Read the model definition and answer for the solid it produces. Units are mm, in the model's axes. A direction names the side the tool comes from. Round coordinates to 2 decimals unless told otherwise and drop trailing zeros. Order: outer loops, then holes, each group sorted by start corner. A loop starts at its lowest first (then second) coordinate and runs counter-clockwise, first axis right, second up. Notation, with made-up numbers: (89, -22) -> (114, -22) arc R21 cw to (114, -18) -> close; hole circle Ø9 at (32, -16.75). An arc over 180 degrees is marked (long way). Answer as a JSON object with one key per item and string values. Group by question number.
Item 1: Section B-B, the plane z = 10.5 is taken. Write down the section's boundary in (x, y), plus the area to 3 significant figures.
Item 2: Consider probe 1 along X at (y, z) = (1.5, -6); probe 2 along Y at (x, z) = (-2.75, 0.5). Determine where each line is inside the solid, lowest interval first. Write a range as from..to.
Item 3: The mould has two halves that part along X. Classify faces 3 (the flat face through (-6, -0.9, 0)), 4 (the flat face through (0, 2.4, 0)), 5 (the flat face through (3.5, 1, 0)), 6 (the flat face through (-8.5, 2, 0)): pulls with the +X half, pulls with the -X half, needs draft (parallel to the pull), parting line crosses it, or undercut.
Item 4: For faces 1 (the flat face through (-3.5, 1, 0)), 2 (the flat face through (0, 3, -15.4)), determine the directions among +Z, -Z, +X, -X, +Y, -Y from which every point of the face is accessible in a straight line to the end or side of a thin tool.
Item 5: Section A-A, the plane y = 0 is taken. Write down the section's boundary in (x, z), plus the area to 3 significant figures.
Item 6: Section C-C, the plane x = -2.25 is taken. Write down the section's boundary in (y, z).
from build123d import *

# Parameters (mm, degrees)
BOSS_EXTRUDE1_DEPTH = 15.4


with BuildPart() as part:
    # Sketch1 → Boss-Extrude1 (new, symmetric)
    with BuildSketch(Plane.XY):
        Polygon((3.5, 2.4), (3.5, -0.9), (8.5, -0.9), (8.5, 5.6), (-8.5, 5.6), (-8.5, -0.9), (-3.5, -0.9), (-3.5, 2.4), align=None)
    extrude(amount=BOSS_EXTRUDE1_DEPTH, both=True)


solid = part.part
Values found:
{
 "1": {"outline": "(-8.5, -0.9) -> (-3.5, -0.9) -> (-3.5, 2.4) -> (3.5, 2.4) -> (3.5, -0.9) -> (8.5, -0.9) -> (8.5, 5.6) -> (-8.5, 5.6) -> close", "area": "87.4 mm2"},
 "2": {"probe 1": "-8.5..-3.5, 3.5..8.5", "probe 2": "2.4..5.6"},
 "3": {"face 3": "needs draft", "face 4": "undercut", "face 5": "undercut", "face 6": "pulls with the -X half"},
 "4": {"face 1": "+Z, -Z, -Y", "face 2": "-Z, +X, -X, +Y, -Y"},
 "5": {"outline": "(-8.5, -15.4) -> (-3.5, -15.4) -> (-3.5, 15.4) -> (-8.5, 15.4) -> close; (3.5, -15.4) -> (8.5, -15.4) -> (8.5, 15.4) -> (3.5, 15.4) -> close", "area": "308 mm2"},
 "6": {"outline": "(2.4, -15.4) -> (5.6, -15.4) -> (5.6, 15.4) -> (2.4, 15.4) -> close"}
}
